Autodesk Inventor part; units mm, degrees
ref_plane "Arbeitsebene1" through (0, 0, 0) normal (-1, 0, 0) x (0, -1, 0)
ref_plane "YZ Plane" through (0, 0, 0) normal (1, 0, 0) x (0, 1, 0)
ref_plane "XZ Plane" through (0, 0, 0) normal (0, 1, 0) x (-1, 0, 0)
sketch "Skizze1" plane through (0, 0, 0) normal (0, 0, 1) x (1, 0, 0)
  line L0 (12, 2) -> (12, 32)
  line L1 (80, 2) -> (80, 32)
  arc A0 (14, 34) -> (12, 32) centre (14, 32) ccw
  arc A1 (80, 32) -> (78, 34) centre (78, 32) ccw
  line L2 (10, 0) -> (0, 0)
  line L3 (82, 0) -> (92, 0)
  arc A2 (80, 2) -> (82, 0) centre (82, 2) ccw
  arc A3 (10, 0) -> (12, 2) centre (10, 2) ccw
  line L4 (78, 34) -> (14, 34)
  dimension "d1" = 30
  dimension "d2" = 30
  dimension "d3" = 2
  dimension "d7" = 2
  dimension "d29" = 2
  dimension "d30" = 2
  dimension "d31" = 92
  dimension "d32" = 10
  dimension "d33" = 10
ref_plane "Arbeitsebene1" through (0, 0, 0) normal (-1, 0, 0) x (0, -1, 0)
sketch "Skizze2" plane through (0, 0, 0) normal (-1, 0, 0) x (0, -1, 0)
  line L0 (-1, 6) -> (1, 6)
  line L1 (1, 6) -> (1, -6)
  line L2 (1, -6) -> (-1, -6)
  line L3 (-1, -6) -> (-1, 6)
  point P0 (0, 0)
  point P1 (1, 0)
  dimension "d15" = 12
  dimension "d16" = 6
  dimension "d17" = 1
  dimension "d18" = 2
sweep "Sweeping1" add profiles "Skizze2" path "Skizze1"
sketch "Skizze4" plane through (0, -1, 6) normal (0, -1, 0) x (1, 0, 0)
  circle A0 centre (5, -6) radius 2
  circle A1 centre (87, -6) radius 2
  line L0 (0, -12) -> (0, 0)
  line L1 (92, -12) -> (92, 0)
  line L2 (92, 0) -> (82, 0)
  point P0 (0, -6)
  dimension "d37" = 4
  dimension "d38" = 4
  dimension "d39" = 5
  dimension "d40" = 5
  dimension "d41" = 6
extrude "Extrusion2" cut sketch "Skizze4" against normal blind 4
fillet "Rundung1" radius 2 4 edges at (92, 0, -6) (92, 0, 6) (0, 0, -6) (0, 0, 6)
equation "\"d1\" = d2"
equation "\"d3\" = d4"
equation "\"d7\" = d4"
properties part number "Handle"
Here's how the part is built. I have some questions about the finished solid (model axes, mm). A direction names the side the tool comes from. Coordinates: 2 decimals unless noted, no trailing zeros. Order: outer loops, then holes, each group sorted by start corner. A loop starts at its lowest first (then second) coordinate and runs counter-clockwise, first axis right, second up. Notation, with made-up numbers: (81.25, -33) -> (123.25, -33) arc R5 cw to (123.25, -25) -> close; hole circle Ø1 at (49, 42). An arc over 180 degrees is marked (long way). Return JSON: item names as keys, results as strings.
1) If we section it at A-A on z = 0: List the corners of the cut face in (x, y) for me, plus the area to 3 significant figures.
Conclusion:
{"outline": "(0, -1) -> (3, -1) -> (3, 1) -> (0, 1) -> close; (7, -1) -> (10, -1) arc R3 ccw to (13, 2) -> (13, 32) arc R1 cw to (14, 33) -> (78, 33) arc R1 cw to (79, 32) -> (79, 2) arc R3 ccw to (82, -1) -> (85, -1) -> (85, 1) -> (82, 1) arc R1 cw to (81, 2) -> (81, 32) arc R3 ccw to (78, 35) -> (14, 35) arc R3 ccw to (11, 32) -> (11, 2) arc R1 cw to (10, 1) -> (7, 1) -> close; (89, -1) -> (92, -1) -> (92, 1) -> (89, 1) -> close", "area": "297 mm²"}
2) I'm going to push flat-ended pins straight in: P1, Ø2.5, axis at x = 5, z = 0, coming from the -Y side; P2, Ø1, axis at y = 16.5, z = 4.5, coming from the +X side; P3, Ø1.5, axis at y = 27.5, z = -3.5, coming from the -X side; P4, Ø3, axis at x = 6, z = 2, coming from the +Y side. Where does each tip first touch, or does it pass through?
Conclusion:
{"P1": "passes through", "P2": "stops at x = 81", "P3": "stops at x = 11", "P4": "stops at y = 1"}
3) If we section it at D-D on x = 8.5: List the corners of the cut face in (y, z) for me.
Conclusion:
{"outline": "(-1, -6) -> (1, -6) -> (1, 6) -> (-1, 6) -> close"}
4) If we section it at B-B on y = 27: List the corners of the cut face in (x, z) for me.
Conclusion:
{"outline": "(11, -6) -> (13, -6) -> (13, 6) -> (11, 6) -> close; (79, -6) -> (81, -6) -> (81, 6) -> (79, 6) -> close"}
5) On a 3-axis mill with a long thin cutter (end or side, diameter ignored), from which of +Z, -Z, +X, -X, +Y, -Y can I reach the whole of each face in a straight line? I mean faces 4 (the flat face through (84.8, 1, 0.1)), 5 (the cylindrical face through (12.1, -0.14, 0.08)), 6 (the flat face through (7.3, 1, 0.1)). Say none if no direction works.
Conclusion:
{"face 4": "+Z, -Z, +X, +Y", "face 5": "+Z, -Z, -Y", "face 6": "+Z, -Z, -X, +Y"}
6) If we section it at C-C on x = 87: List the corners of the cut face in (y, z) for me.
Conclusion:
{"outline": "(-1, -6) -> (1, -6) -> (1, -2) -> (-1, -2) -> close; (-1, 2) -> (1, 2) -> (1, 6) -> (-1, 6) -> close"}
7) If I drill on probe 1 along Z at (x, y) = (5, -0.2); probe 2 along X at (y, z) = (31, 1.25); probe 3 along Y at (x, z) = (77, 4.5), over which ranges is the centre line in solid material (lowest first)?
Conclusion:
{"probe 1": "z = -6 to -2, 2 to 6", "probe 2": "x = 11 to 13, 79 to 81", "probe 3": "y = 33 to 35"}
8) Thinking about a two-plate mould opening in Z: for faces 1 (the cylindrical face through (88.908, -0.014, 0.601)), 2 (the cylindrical face through (91.4, -0.01, -5.43)), 3 (the cylindrical face through (79.86, -0.1, 0.08)), which applies, +Z half, -Z half, draft (parallel to the pull), parting line (faces both ways), or undercut?
Conclusion:
{"face 1": "undercut", "face 2": "-Z half", "face 3": "draft"}
